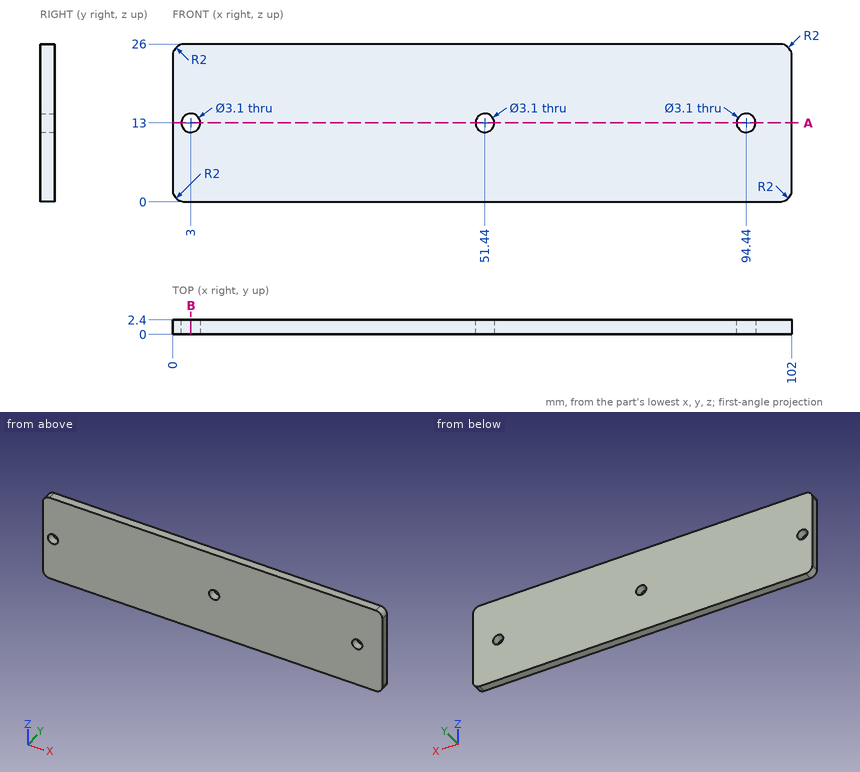
The figure shows three views and two pictorial views of one solid part (mm, origin at its lowest corner). Answer the questions. Coordinates: 2 decimals unless noted, no trailing zeros. Write each loop counter-clockwise with the first axis right and the second up, starting at its lowest first coordinate (ties: lowest second). Pieces come first, ordered by that corner, then holes.
1. Consider line 1 along X through (y, z) = (1.15, 12.75); line 2 along Z through (x, y) = (3, 1.7); line 3 along X through (y, z) = (1.2, 24.25). Determine where each line is inside the solid, lowest interval first.
Results list:
line 1: x = 0 to 1.47, 4.53 to 49.91, 52.97 to 92.91, 95.97 to 102
line 2: z = 0 to 11.45, 14.55 to 26
line 3: x = 0.02 to 101.98
2. The part is cut by section A-A, the plane z = 13. Write down the section's boundary in (x, y).
Results list:
outline: (0, 0) - (1.45, 0) - (1.45, 2.4) - (0, 2.4) - close; (4.55, 0) - (49.89, 0) - (49.89, 2.4) - (4.55, 2.4) - close; (52.99, 0) - (92.89, 0) - (92.89, 2.4) - (52.99, 2.4) - close; (95.99, 0) - (102, 0) - (102, 2.4) - (95.99, 2.4) - close
3. Flat-ended cylindrical pins translate along their axes: pin 1 (4 mm diameter, centred on x = 94.44, z = 13, fed in from +Y); pin 2 (1.9 mm diameter, centred on x = 51.44, z = 13, fed in from -Y). Find the tip coordinate at first contact, or state that the pin passes through.
Results list:
pin 1: stops at y = 2.4
pin 2: passes through
4. The part is cut by section B-B, the plane x = 3. Write down the section's boundary in (y, z).
Results list:
outline: (0, 0) - (2.4, 0) - (2.4, 11.45) - (0, 11.45) - close; (0, 14.55) - (2.4, 14.55) - (2.4, 26) - (0, 26) - close
